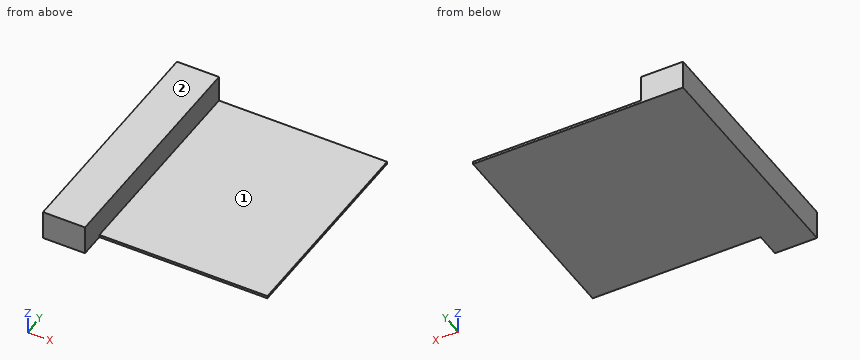
from build123d import *

# Parameters (mm, degrees)
F0_W     = 100
F0_H     = 100
F1_DEPTH = 1.2
F2_W     = 20
F2_H     = 100
F3_DEPTH = 12.7
F5_DEPTH = 12


with BuildPart() as f1:
    # F0 (on Top) → F1 (new body)
    with BuildSketch(Plane.XY):
        Rectangle(F0_W, F0_H)
    extrude(amount=F1_DEPTH)

    # F2 (on face) → F3 (join)
    with BuildSketch(Plane.XY.offset(1.2)):
        with Locations((-40, 0)):
            Rectangle(F2_W, F2_H)
    extrude(amount=F3_DEPTH)

    # F4 (on face) → F5 (join)
    with BuildSketch(Plane.XZ.offset(50)):
        Polygon((-30, 13.9), (-50, 13.9), (-50, 0), (-30, 0), (-30, 1.2), align=None)
    extrude(amount=F5_DEPTH)


solid = f1.part
The model under review builds one solid part; all positions refer to its coordinate system, in mm. Face numbers are marked on the shaded views. A direction names the side the tool comes from. Give positions to 0.01 mm unless a question says otherwise; leave off trailing zeros. Order: outer loops, then holes, each group sorted by start corner. A loop starts at its lowest first (then second) coordinate and runs counter-clockwise, first axis right, second up. Notation, with made-up numbers: M 25,-35.75 L 79,-35.75 A23 cw 79,-13.75 Z; hole C -37,10 d7. An arc over 180 degrees is marked long. Answer in a Markdown table with one row per item. Add a question column.
1. Add section C-C on x = -1. State the section outline as (y, z) points.
2. Machinability: for the marked faces 1 and 2, which of the approach directions +Z, -Z, +X, -X, +Y, -Y give a long, thin tool a straight path to every point of the face, cutting with its end or side? Answer none if there is none.
3. For pin 1 Ø5 at (x, z) = (38.5, 3) entering from -Y; pin 2 Ø8 at (x, y) = (-14, -14) entering from +Z; pin 3 Ø4 at (y, z) = (-20, 9.5) entering from +X, all flat-tipped, find the tip position at first contact; note any pin that passes through.
4. Add section A-A on z = 12. State the section outline as (x, y) points.
5. To check wall thickness, follow line 1 along X through (y, z) = (-4.5, 10.5); line 2 along Z through (x, y) = (11.5, -12); line 3 along Y through (x, z) = (21, 1). State the ranges of each line that lie inside material, in increasing order.
6. Add section B-B on y = 19. State the section outline as (x, z) points.
The answers:
| question | item | result |
|---|---|---|
| 1 | outline | M -50,0 L 50,0 L 50,1.2 L -50,1.2 Z |
| 2 | face 1 | +Z, +X, +Y, -Y |
| 2 | face 2 | +Z, +X, -X, +Y, -Y |
| 3 | pin 1 | y = -50 |
| 3 | pin 2 | z = 1.2 |
| 3 | pin 3 | x = -30 |
| 4 | outline | M -50,-62 L -30,-62 L -30,50 L -50,50 Z |
| 5 | line 1 | -50 to -30 |
| 5 | line 2 | 0 to 1.2 |
| 5 | line 3 | -50 to 50 |
| 6 | outline | M -50,0 L 50,0 L 50,1.2 L -30,1.2 L -30,13.9 L -50,13.9 Z |
